For this review, take the finished solid that the model builds, in its own axes (mm). Face numbers are marked on the shaded views. A direction names the side the tool comes from. Round coordinates to 2 decimals unless told otherwise and drop trailing zeros. Order: outer loops, then holes, each group sorted by start corner. A loop starts at its lowest first (then second) coordinate and runs counter-clockwise, first axis right, second up. Notation, with made-up numbers: (36.5, 35.25) -> (72.5, 35.25) arc R17 ccw to (72.5, 62.25) -> close; hole circle Ø6 at (17.25, 46). An arc over 180 degrees is marked (long way). Use a Markdown table: item, result. Add a question column.
1) Draft analysis for pull direction Z (two halves, no side actions). For the marked faces 6, 7, 8 and 9, state which applies: pulls with the +Z half, pulls with the -Z half, needs draft (parallel to the pull), parting line crosses it, or undercut.
2) Consider section C-C (y = -217). State the section outline as (x, z) points.
3) Clearance check with flat-ended pins moving along their axes: P1, Ø10, axis at x = -79.5, z = -520.5, coming from the +Y side; P2, Ø5, axis at x = 150, y = -52.5, coming from the +Z side; P3, Ø10, axis at x = -22.5, y = -315.5, coming from the +Z side. State where each tip first meets the part, or that it passes through.
4) Consider section D-D (y = -418.5). State the section outline as (x, z) points.
5) Machinability: for the marked faces 1, 2, 3, 4 and 5, which of the approach directions +Z, -Z, +X, -X, +Y, -Y give a long, thin tool a straight path to every point of the face, cutting with its end or side? Answer none if there is none.
6) Wall thickness on line 1 along Z through (x, y) = (0, -45); line 2 along Y through (x, z) = (225.5, -212); line 3 along Z through (x, y) = (0, -437.5): over which ranges is each line inside the solid? List them lowest first. Write a range as [from, to].
7) Consider section A-A (z = 0). State the section outline as (x, y) points, plus the area to 3 significant figures.
8) Consider section B-B (x = 0). State the section outline as (y, z) points.
```python
from build123d import *

# Parameters (mm, degrees)
F0_R     = 125
F0_R_2   = 50
F1_DEPTH = 460
F2_W     = 260
F2_H     = 420
F3_DEPTH = 550.001
F4_W     = 550
F4_H     = 710
F5_DEPTH = 30
F6_W     = 550
F6_H     = 710
F7_DEPTH = 30


with BuildPart() as f1:
    # F0 (on Front) → F1 (new body)
    with BuildSketch(Plane.XZ):
        Polygon((135, 120), (-135, 120), (-275, -20), (-275, -120), (-275, -900), (-125, -1050), (125, -1050), (275, -900), (275, -120), (275, -20), align=None)
        with Locations((0, -750)):
            Circle(F0_R, mode=Mode.SUBTRACT)
        Circle(F0_R_2, mode=Mode.SUBTRACT)
    extrude(amount=F1_DEPTH)

    # F2 (on face) → F3 (cut, through all)
    with BuildSketch(Plane.YZ.offset(275)):
        with Locations((-230, -20)):
            Rectangle(F2_W, F2_H)
    extrude(amount=-F3_DEPTH, mode=Mode.SUBTRACT)

    # F4 (on face) → F5 (cut)
    with BuildSketch(Plane(origin=(0, 0, 0), x_dir=(-1, 0, 0), z_dir=(0, 1, 0))):
        with Locations((0, -695)):
            Rectangle(F4_W, F4_H)
    extrude(amount=-F5_DEPTH, mode=Mode.SUBTRACT)

    # F6 (on face) → F7 (cut)
    with BuildSketch(Plane.XZ.offset(460)):
        with Locations((0, -695)):
            Rectangle(F6_W, F6_H)
    extrude(amount=-F7_DEPTH, mode=Mode.SUBTRACT)


solid = f1.part
```
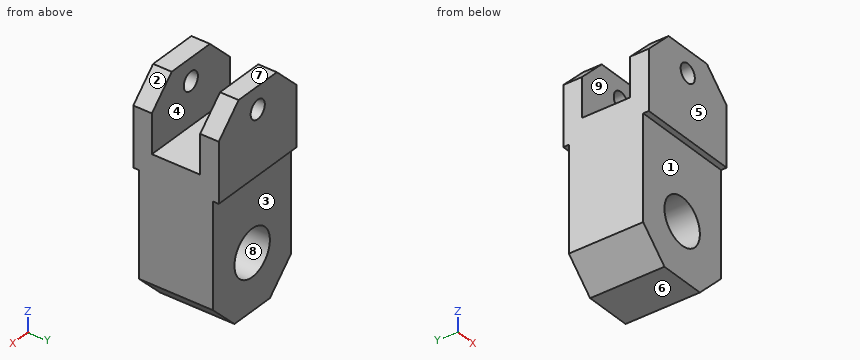
Results list:
| question | item | result |
|---|---|---|
| 1 | face 6 | pulls with the -Z half |
| 1 | face 7 | pulls with the +Z half |
| 1 | face 8 | undercut |
| 1 | face 9 | needs draft |
| 2 | outline | (-275, -900) -> (-125, -1050) -> (125, -1050) -> (275, -900) -> (275, -230) -> (-275, -230) -> close; hole circle Ø250 at (0, -750) |
| 3 | P1 | y = -30 |
| 3 | P2 | z = 107.5 |
| 3 | P3 | z = -230 |
| 4 | outline | (-275, -900) -> (-125, -1050) -> (125, -1050) -> (275, -900) -> (275, -20) -> (135, 120) -> (-135, 120) -> (-275, -20) -> close; hole circle Ø250 at (0, -750); hole circle Ø100 at (0, 0) |
| 5 | face 1 | -Z, +X, -X, -Y |
| 5 | face 2 | +Z, +X, +Y, -Y |
| 5 | face 3 | -Z, +X, -X, +Y |
| 5 | face 4 | +Z, +X, -X |
| 5 | face 5 | +Z, -Z, +X, -X, -Y |
| 6 | line 1 | [-1050, -875], [-625, -50], [50, 120] |
| 6 | line 2 | [-460, -360], [-100, 0] |
| 6 | line 3 | [-340, -50], [50, 120] |
| 7 | outline | (-255, -460) -> (-50, -460) -> (-50, -360) -> (-255, -360) -> close; (-255, -100) -> (-50, -100) -> (-50, 0) -> (-255, 0) -> close; (50, -460) -> (255, -460) -> (255, -360) -> (50, -360) -> close; (50, -100) -> (255, -100) -> (255, 0) -> (50, 0) -> close |
| 7 | area | 82,000 mm2 |
| 8 | outline | (-460, -340) -> (-430, -340) -> (-430, -625) -> (-30, -625) -> (-30, -340) -> (0, -340) -> (0, -50) -> (-100, -50) -> (-100, -230) -> (-360, -230) -> (-360, -50) -> (-460, -50) -> close; (-460, 50) -> (-360, 50) -> (-360, 120) -> (-460, 120) -> close; (-430, -1050) -> (-30, -1050) -> (-30, -875) -> (-430, -875) -> close; (-100, 50) -> (0, 50) -> (0, 120) -> (-100, 120) -> close |
